Model file for the job. Use its own axes, mm. A direction names the side the tool comes from. Give positions to 0.01 mm unless a question says otherwise; leave off trailing zeros. Loops run counter-clockwise (first coordinate to the right, second up) from the corner with the lowest first, then second, coordinate; pieces in that order, holes last. Notation, with made-up numbers: M -25.75,66.25 L 25.25,66.25 A14 ccw 25.25,86.25 Z; hole C -6,84 d11. An arc over 180 degrees is marked long. Answer in a Markdown table with one row per item.
```python
from build123d import *

# Parameters (mm, degrees)
SKETCH1_R           = 75
BOSS_EXTRUDE1_DEPTH = 110
SKETCH3_W           = 100
SKETCH3_H           = 100
BOSS_EXTRUDE2_DEPTH = 70
SKETCH4_R           = 55
CUT_EXTRUDE1_DEPTH  = 42


with BuildPart() as part:
    # Sketch1 → Boss-Extrude1 (new body)
    with BuildSketch(Plane.XY):
        Circle(SKETCH1_R)
    extrude(amount=BOSS_EXTRUDE1_DEPTH)

    # Sketch3 → Boss-Extrude2 (add)
    with BuildSketch(Plane(origin=(0, 0, 0), x_dir=(-1, 0, 0), z_dir=(0, 0, -1))):
        Rectangle(SKETCH3_W, SKETCH3_H)
    extrude(amount=BOSS_EXTRUDE2_DEPTH)

    # Sketch4 → Cut-Extrude1 (cut)
    with BuildSketch(Plane.XY.offset(110)):
        Circle(SKETCH4_R)
    extrude(amount=-CUT_EXTRUDE1_DEPTH, mode=Mode.SUBTRACT)


solid = part.part
```
(1) Wall check: L1, parallel to Y at x = 0, z = 87; L2, parallel to Z at x = -65, y = -20.5; L3, parallel to Y at x = 17, z = -28. Give the ranges that are in metal, low to high.
Established:
| item | result |
|---|---|
| L1 | y = -75 to -55, 55 to 75 |
| L2 | z = 0 to 110 |
| L3 | y = -50 to 50 |
(2) Saw through at B-B, the plane z = 92. Give the cut face in (x, y).
Established:
| item | result |
|---|---|
| outline | C 0,0 d150; hole C 0,0 d110 |
(3) Flat gauge pins, fed straight in: P1, Ø10, axis at x = -20, z = 49, coming from the -Y side; P2, Ø3, axis at y = 37, z = -51.5, coming from the +X side; P3, Ø1.5, axis at x = 4.5, z = 51, coming from the +Y side. Where does each tip first touch, or does it go through?
Established:
| item | result |
|---|---|
| P1 | stops at y = -73.48 |
| P2 | stops at x = 50 |
| P3 | stops at y = 74.91 |
(4) Saw through at D-D, the plane z = -58.5. Give the cut face in (x, y).
Established:
| item | result |
|---|---|
| outline | M -50,-50 L 50,-50 L 50,50 L -50,50 Z |
(5) Which spindle directions (+Z, -Z, +X, -X, +Y, -Y) get a long thin tool onto all of the face, cutting with end or side? Do faces 4 (the cylindrical face through (-9.764, 74.362, 54.23)), 5 (the cylindrical face through (-11.923, -53.692, 89.294)), 6 (the flat face through (1, 50, -35)), 7 (the flat face through (1, -50, -35)), 8 (the flat face through (-50, -1, -35)). Say none if no direction does.
Established:
| item | result |
|---|---|
| face 4 | +Z, -Z |
| face 5 | +Z |
| face 6 | -Z, +X, -X, +Y |
| face 7 | -Z, +X, -X, -Y |
| face 8 | -Z, -X, +Y, -Y |
(6) Saw through at A-A, the plane y = 0. Give the cut face in (x, z), and give its area (3 significant figures).
Established:
| item | result |
|---|---|
| outline | M -75,0 L -50,0 L -50,-70 L 50,-70 L 50,0 L 75,0 L 75,110 L 55,110 L 55,68 L -55,68 L -55,110 L -75,110 Z |
| area | 18,900 mm2 |
(7) Mould opens along X. For faces 1 (the flat face through (-50.4, -5.2, 0)), 2 (the flat face through (-1, 1, 68)), 3 (the flat face through (50, -1, -35)) say: pulls with the +X half, pulls with the -X half, needs draft (parallel to the pull), parting line crosses it, or undercut.
Established:
| item | result |
|---|---|
| face 1 | needs draft |
| face 2 | undercut |
| face 3 | pulls with the +X half |
